from build123d import *

# Parameters (mm, degrees)
F0_W     = 30.743243
F0_H     = 41.621625
F1_DEPTH = 3


with BuildPart() as f1:
    # F0 (on Front) → F1 (new body)
    with BuildSketch(Plane.XZ):
        with Locations((31.689193, -31.925679)):
            Rectangle(F0_W, F0_H)
        Polygon((20.574326, -48.952702), (20.574326, -14.268018), (42.961713, -14.268018), (42.961713, -48.952702), (29.87613, -20.731982), align=None, mode=Mode.SUBTRACT)
    extrude(amount=F1_DEPTH)


solid = f1.part
Work out the finished part from the listing and answer in its coordinate system (mm). A direction names the side the tool comes from. Give positions to 0.01 mm unless a question says otherwise; leave off trailing zeros. Loops run counter-clockwise (first coordinate to the right, second up) from the corner with the lowest first, then second, coordinate; pieces in that order, holes last. Notation, with made-up numbers: (34.5, 45) -> (81.5, 45) arc R23 ccw to (81.5, 55) -> close; hole circle Ø4 at (18, 31). An arc over 180 degrees is marked (long way). Use a Markdown table: item, result. Add a question column.
1) The part is cut by section D-D, the plane z = -44.5. Determine the outline of the cut face in (x, y), plus the area to 3 significant figures.
2) This flat-tipped pin is pushed along its axis until it touches: P1, Ø1.5, axis at x = 28.5, z = -35, coming from the +Y side. Where does it stop, or does it pass through?
3) The part is cut by section A-A, the plane z = -15.5. Determine the outline of the cut face in (x, y), plus the area to 3 significant figures.
4) Which of the six approach directions +Z, -Z, +X, -X, +Y, -Y give full straight-line access (tool end or side, diameter ignored) to faces 4 (the flat face through (16.318, -1, -32)), 5 (the flat face through (42.962, -1, -31))?
5) The part is cut by section B-B, the plane y = -0.8. Determine the outline of the cut face in (x, z), plus the area to 3 significant figures.
6) Consider line 1 along X through (y, z) = (-0.5, -19); line 2 along X through (y, z) = (-2.35, -40.5); line 3 along X through (y, z) = (-2, -40). Determine where each line is inside the solid, lowest interval first.
7) For a pull along Z with two mould halves and no side action, classify faces 1 (the flat face through (31, -3, -36)), 2 (the flat face through (31, -1, -52.736)), 3 (the flat face through (36.51, -1.48, -35.04)) as +Z half, -Z half, draft (parallel to the pull), parting line (faces both ways), or undercut.
8) The part is cut by section C-C, the plane x = 22. Determine the outline of the cut face in (y, z).
Reported:
| question | item | result |
|---|---|---|
| 1 | outline | (16.32, -3) -> (20.57, -3) -> (20.57, 0) -> (16.32, 0) -> close; (22.04, -3) -> (40.9, -3) -> (40.9, 0) -> (22.04, 0) -> close; (42.96, -3) -> (47.06, -3) -> (47.06, 0) -> (42.96, 0) -> close |
| 1 | area | 81.6 mm^2 |
| 2 | P1 | stops at y = 0 |
| 3 | outline | (16.32, -3) -> (20.57, -3) -> (20.57, 0) -> (16.32, 0) -> close; (42.96, -3) -> (47.06, -3) -> (47.06, 0) -> (42.96, 0) -> close |
| 3 | area | 25.1 mm^2 |
| 4 | face 4 | +Z, -Z, -X, +Y, -Y |
| 4 | face 5 | +Y, -Y |
| 5 | outline | (16.32, -52.74) -> (47.06, -52.74) -> (47.06, -11.11) -> (16.32, -11.11) -> close; hole (20.57, -48.95) -> (29.88, -20.73) -> (42.96, -48.95) -> (42.96, -14.27) -> (20.57, -14.27) -> close |
| 5 | area | 819 mm^2 |
| 6 | line 1 | x = 16.32 to 20.57, 42.96 to 47.06 |
| 6 | line 2 | x = 16.32 to 20.57, 23.36 to 39.04, 42.96 to 47.06 |
| 6 | line 3 | x = 16.32 to 20.57, 23.53 to 38.81, 42.96 to 47.06 |
| 7 | face 1 | draft |
| 7 | face 2 | -Z half |
| 7 | face 3 | undercut |
| 8 | outline | (-3, -52.74) -> (0, -52.74) -> (0, -44.63) -> (-3, -44.63) -> close; (-3, -14.27) -> (0, -14.27) -> (0, -11.11) -> (-3, -11.11) -> close |
